Could you check a few things on this model? Use its own coordinates, in mm. Face numbers are marked on the shaded views. A direction names the side the tool comes from. Coordinates: 2 decimals unless noted, no trailing zeros. Loops run counter-clockwise (first coordinate to the right, second up) from the corner with the lowest first, then second, coordinate; pieces in that order, holes last. Notation, with made-up numbers: (6, 9.5) - (29, 9.5) arc R26 cw to (29, 32.5) - close; hole circle Ø1 at (16, -12.75). An arc over 180 degrees is marked (long way). One line per question, with ' | ' between items. Start each with the question number.
1. I want a section at A-A, the plane x = -376. Write out the boundary of the cut face in (y, z).
2. We'd pull the mould along Y, two halves only. Please class the marked faces 1, 2 and 3: pulls with the +Y half, pulls with the -Y half, needs draft (parallel to the pull), parting line crosses it, or undercut.
3. I want a section at C-C, the plane z = 76. Write out the boundary of the cut face in (x, y).
4. Which directions (+Z, -Z, +X, -X, +Y, -Y) give clear straight access to the entire face, cutting with the end or side of a thin tool? Please do the marked faces 4, 5 and 6.
5. Please list where these lines run through material, in increasing order: L1, parallel to Y at x = -221, z = 8.5; L2, parallel to X at y = 9, z = 67; L3, parallel to Y at x = -211, z = 36.5. Write a range as [from, to].
6. I want a section at D-D, the plane z = -27. Write out the boundary of the cut face in (x, y), then the cut area to 3 significant figures.
7. I want a section at B-B, the plane y = 186. Write out the boundary of the cut face in (x, z).
8. I'm going to push flat-ended pins straight in: P1, Ø1.5, axis at x = -342.5, y = 93, coming from the +Z side (3 decimals); P2, Ø22, axis at y = 146, z = 38, coming from the +X side; P3, Ø10, axis at x = -118.5, z = 76.5, coming from the +Y side; P4, Ø6, axis at x = -145.5, z = -52.5, coming from the +Y side. Where does each tip first touch, or does it pass through?
from build123d import *

# Parameters (mm, degrees)
BOSS_EXTRUDE2_DEPTH      = 6.35
BOSS_EXTRUDE3_DEPTH      = 254
BOSS_EXTRUDE3_DEPTH_BACK = 6.35
BOSS_EXTRUDE4_DEPTH      = 254
BOSS_EXTRUDE4_DEPTH_BACK = 6.35
BOSS_EXTRUDE5_DEPTH      = 133.35
BOSS_EXTRUDE6_DEPTH      = 6.35
BOSS_EXTRUDE8_DEPTH      = 6.35
BOSS_EXTRUDE9_DEPTH      = 6.35
BOSS_EXTRUDE10_DEPTH     = 6.35


with BuildPart() as part:
    # 3DSketch1 → Boss-Extrude2 (new body)
    with BuildSketch(Plane(origin=(0, 1.332156405, 65.630699338), x_dir=(0, 0.9561985348142941, -0.2927189129847902), z_dir=(-1, 0, 0))):
        Polygon((0, 0), (33.457771754, 109.293492529), (55.888968865, 121.2099264), (249.70876595, 0), (242.27370556, -24.287442784), (17.363491096, -32.684601412), align=None)
    extrude(amount=BOSS_EXTRUDE2_DEPTH)

    # Sketch2 → Boss-Extrude3 (add, two sides: drawn at the far end of the back side and taken through both)
    with BuildSketch(Plane.ZY.offset(6.35).offset(-BOSS_EXTRUDE3_DEPTH_BACK)):
        Polygon((-61.445059615, 14.107915358), (-48.669300662, 1.332156405), (65.630699338, 1.332156405), (88.807649546, 24.509106613), (86.118065358, 32.250379724), (89.717035392, 33.500785537), (91.80104508, 27.502502147), (97.799328469, 29.586511835), (95.715318781, 35.584795224), (98.114632137, 36.4183991), (101.101183052, 27.822383999), (68.260955459, -5.017843595), (-51.299556783, -5.017843595), (-76.823169583, 20.505769205), (-74.800118363, 28.055899142), (-71.119940965, 27.069798581), (-72.763441901, 20.936169584), (-66.629812904, 19.292668647), (-64.986311968, 25.426297644), (-58.852682971, 23.782796708), align=None)
    extrude(amount=BOSS_EXTRUDE3_DEPTH + BOSS_EXTRUDE3_DEPTH_BACK)

    # Sketch4 → Boss-Extrude4 (add, two sides: drawn at the far end of the back side and taken through both)
    with BuildSketch(Plane.ZY.offset(6.35).offset(-BOSS_EXTRUDE4_DEPTH_BACK)):
        Polygon((-0.889775448, 240.103312537), (13.902816842, 240.103312537), (16.42126046, 232.854623335), (20.020230494, 234.105029148), (17.936220806, 240.103312537), (22.024731964, 241.523801752), (24.108741651, 235.525518362), (26.508055007, 236.359122237), (23.000986566, 246.453312537), (-16.280707815, 246.453312537), (-18.921086525, 236.599285038), (-15.240909127, 235.613184476), (-13.597408191, 241.746813473), (-7.463779194, 240.103312537), (-9.10728013, 233.96968354), (-2.973651133, 232.326182604), align=None)
    extrude(amount=BOSS_EXTRUDE4_DEPTH + BOSS_EXTRUDE4_DEPTH_BACK)

    # Sketch5 → Boss-Extrude5 (add)
    with BuildSketch(Plane.ZY.offset(260.35)):
        Polygon((-68.52756432, 12.210163942), (-51.299556783, -5.017843595), (68.260955459, -5.017843595), (101.101183052, 27.822383999), (98.114632137, 36.4183991), (95.715318781, 35.584795224), (97.799328469, 29.586511835), (91.80104508, 27.502502147), (89.717035392, 33.500785537), (86.118065358, 32.250379724), (88.807649546, 24.509106613), (65.630699338, 1.332156405), (-48.669300662, 1.332156405), (-61.445059615, 14.107915358), (-0.889775448, 240.103312537), (13.902816842, 240.103312537), (16.42126046, 232.854623335), (20.020230494, 234.105029148), (17.936220806, 240.103312537), (22.024731964, 241.523801752), (24.108741651, 235.525518362), (26.508055007, 236.359122237), (23.000986566, 246.453312537), (-5.762301822, 246.453312537), align=None)
    extrude(amount=BOSS_EXTRUDE5_DEPTH)

    # Sketch7 → Boss-Extrude6 (add)
    with BuildSketch(Plane.ZY.offset(260.35)):
        Polygon((-16.280707815, 246.453312537), (-76.823169583, 20.505769205), (-68.52756432, 12.210163942), (-5.762301822, 246.453312537), align=None)
    extrude(amount=BOSS_EXTRUDE6_DEPTH)

    # Sketch9 → Boss-Extrude8 (add)
    with BuildSketch(Plane(origin=(-260.35, 0, 0), x_dir=(0, 0, -1), z_dir=(1, 0, 0))):
        Polygon((15.240909127, 235.613184476), (71.119940965, 27.069798581), (74.800118363, 28.055899142), (18.921086525, 236.599285038), align=None)
        Polygon((2.973651133, 232.326182604), (9.10728013, 233.96968354), (64.986311968, 25.426297644), (58.852682971, 23.782796708), align=None)
    extrude(amount=BOSS_EXTRUDE8_DEPTH)

    # Sketch11 → Boss-Extrude9 (add)
    with BuildSketch(Plane.ZY.offset(393.7)):
        Polygon((23.000986566, 246.453312537), (101.101183052, 27.822383999), (68.260955459, -5.017843595), (-51.299556783, -5.017843595), (-68.52756432, 12.210163942), (-5.762301822, 246.453312537), align=None)
    extrude(amount=BOSS_EXTRUDE9_DEPTH)

    # Sketch12 → Boss-Extrude10 (add)
    with BuildSketch(Plane(origin=(-393.7, 0, 0), x_dir=(0, 0, -1), z_dir=(1, 0, 0))):
        Polygon((-24.108741651, 235.525518362), (-26.508055007, 236.359122237), (-98.114632137, 36.4183991), (-95.715318781, 35.584795224), align=None)
        Polygon((-20.020230494, 234.105029148), (-16.42126046, 232.854623335), (-86.118065358, 32.250379724), (-89.717035392, 33.500785537), align=None)
    extrude(amount=BOSS_EXTRUDE10_DEPTH)


solid = part.part
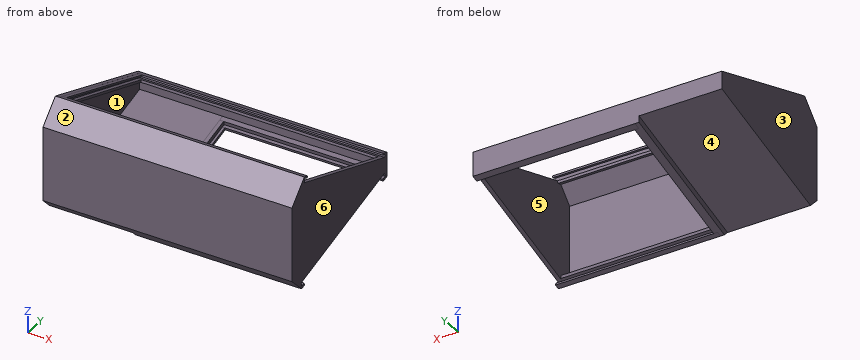
Results are:
1) outline: (-5.02, -51.3) - (12.21, -68.53) - (246.45, -5.76) - (246.45, 23) - (236.36, 26.51) - (235.53, 24.11) - (241.52, 22.02) - (240.1, 17.94) - (234.11, 20.02) - (232.85, 16.42) - (240.1, 13.9) - (240.1, -0.89) - (14.11, -61.45) - (1.33, -48.67) - (1.33, 65.63) - (24.51, 88.81) - (32.25, 86.12) - (33.5, 89.72) - (27.5, 91.8) - (29.59, 97.8) - (35.58, 95.72) - (36.42, 98.11) - (27.82, 101.1) - (-5.02, 68.26) - close
2) face 1: undercut | face 2: pulls with the -Y half | face 3: needs draft
3) outline: (-400.05, 2.72) - (0, 2.72) - (0, 72.98) - (-6.35, 72.98) - (-6.35, 11.7) - (-393.7, 11.7) - (-393.7, 61.37) - (-387.35, 61.37) - (-387.35, 72.98) - (-393.7, 72.98) - (-393.7, 90.63) - (-387.35, 90.63) - (-387.35, 98.17) - (-393.7, 98.17) - (-393.7, 98.09) - (-400.05, 98.09) - close
4) face 4: -Z, -X, +Y | face 5: none | face 6: +Z, -Z, +X, +Y, -Y
5) L1: y = [-5.02, 1.33], [240.1, 246.45] | L2: x = [-400.05, -393.7], [-6.35, 0] | L3: y = [-5.02, 1.33]
6) outline: (-400.05, -5.02) - (0, -5.02) - (0, 167.19) - (-6.35, 167.19) - (-6.35, 1.33) - (-393.7, 1.33) - (-393.7, 142.66) - (-254, 142.66) - (-254, 167.19) - (-260.35, 167.19) - (-260.35, 191.73) - (-254, 191.73) - (-254, 206.45) - (-266.7, 206.45) - (-266.7, 167.19) - (-400.05, 167.19) - close | area: 8,420 mm2
7) outline: (-400.05, -21.96) - (-266.7, -21.96) - (-266.7, -32.48) - (-254, -32.48) - (-254, -28.53) - (-260.35, -28.53) - (-260.35, -21.96) - (-254, -21.96) - (-254, -15.39) - (-393.7, -15.39) - (-393.7, 32.7) - (-387.35, 32.7) - (-387.35, 36.73) - (-393.7, 36.73) - (-393.7, 41.85) - (-387.35, 41.85) - (-387.35, 44.54) - (-393.7, 44.54) - (-393.7, 44.6) - (-400.05, 44.6) - close; (-6.35, -21.96) - (0, -21.96) - (0, 36.73) - (-6.35, 36.73) - close
8) P1: stops at z = -40.105 | P2: stops at x = 0 | P3: stops at y = 17.2 | P4: stops at y = 8.16
